Verification items for this drawing (mm, ordinates from the low corner). Round coordinates to 2 decimals unless told otherwise and drop trailing zeros. Order: outer loops, then holes, each group sorted by start corner. A loop starts at its lowest first (then second) coordinate and runs counter-clockwise, first axis right, second up. Notation, with made-up numbers: (59.25, 64) - (83.25, 64) arc R25 ccw to (83.25, 78) - close; hole circle Ø8 at (65, 26.5). An arc over 180 degrees is marked (long way). One line per question, with ' | ' between items. Start each with the question number.
Q1. Gauge pin test, flat ends, axial feed: P1, Ø1, axis at y = 1, z = 81.5, coming from the +X side; P2, Ø3.5, axis at x = 95.5, z = 6, coming from the -Y side; P3, Ø0.6, axis at y = 1, z = 81, coming from the -X side. Record the tip position at first contact, or that the pin passes through.
Q2. Sectioned sample at B-B, the plane x = 5.5. Enter the section's corners in (y, z), then the cut area to 3 significant figures.
Q3. Material ranges on line 1 along X through (y, z) = (1.1, 6); line 2 along X through (y, z) = (1.4, 6.5); line 3 along Z through (x, y) = (5.5, 1.35), recorded low to high.
Q4. Sectioned sample at A-A, the plane y = 0.45. Enter the section's corners in (x, z), then the cut area to 3 significant figures.
Q5. Sectioned sample at C-C, the plane z = 6. Enter the section's corners in (x, y).
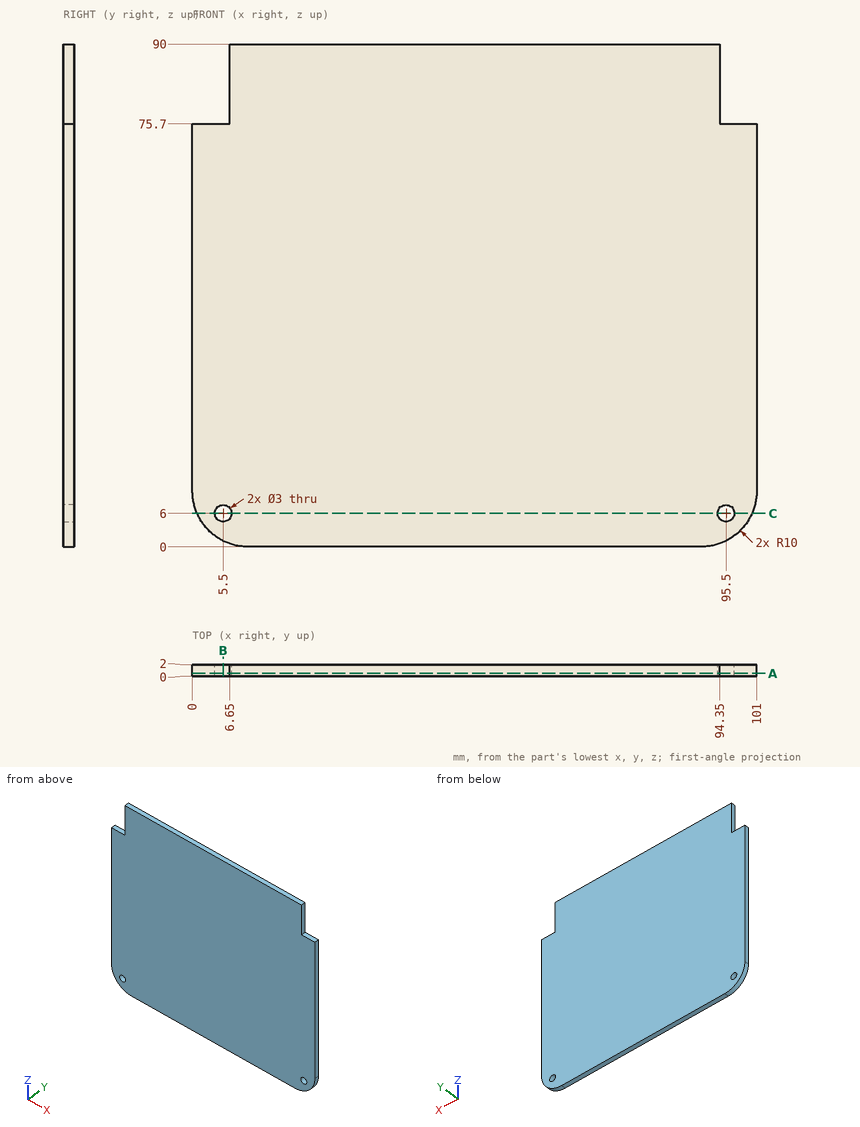
Determined:
1) P1: stops at x = 94.35 | P2: stops at y = 0 | P3: stops at x = 6.65
2) outline: (0, 1.07) - (2, 1.07) - (2, 4.5) - (0, 4.5) - close; (0, 7.5) - (2, 7.5) - (2, 75.7) - (0, 75.7) - close | area: 143 mm2
3) line 1: x = 0.83 to 4, 7 to 94, 97 to 100.17 | line 2: x = 0.63 to 4.09, 6.91 to 94.09, 96.91 to 100.37 | line 3: z = 1.07 to 4.5, 7.5 to 75.7
4) outline: (0, 10) arc R10 ccw to (10, 0) - (91, 0) arc R10 ccw to (101, 10) - (101, 75.7) - (94.35, 75.7) - (94.35, 90) - (6.65, 90) - (6.65, 75.7) - (0, 75.7) - close; hole circle Ø3 at (5.5, 6); hole circle Ø3 at (95.5, 6) | area: 8,840 mm2
5) outline: (0.83, 0) - (4, 0) - (4, 2) - (0.83, 2) - close; (7, 0) - (94, 0) - (94, 2) - (7, 2) - close; (97, 0) - (100.17, 0) - (100.17, 2) - (97, 2) - close
